Source: CAD feature listing. Evaluate the final solid. Frame: model axes, mm. A direction names the side the tool comes from. Round coordinates to 2 decimals unless told otherwise and drop trailing zeros. Loops run counter-clockwise (first coordinate to the right, second up) from the corner with the lowest first, then second, coordinate; pieces in that order, holes last. Notation, with made-up numbers: M -12,15 L 40,15 A23 cw 40,52 Z; hole C 13,67.5 d1. An arc over 180 degrees is marked long. Answer as a JSON object with one key per item and string values.
from build123d import *

# Parameters (mm, degrees)
ESQUISSE1_R                  = 4.1
BOSS_EXTRU_1_DEPTH           = 5
ESQUISSE2_R                  = 8.25
ENL_V_MAT_EXTRU_1_DEPTH      = 3
ESQUISSE4_W                  = 3
ESQUISSE4_H                  = 5
ENL_V_MAT_EXTRU_2_DEPTH      = 2
BOSS_EXTRU_2_DEPTH           = 5
ENL_V_MAT_EXTRU_4_DEPTH      = 5
ESQUISSE8_R                  = 2.75
ENL_V_MAT_EXTRU_5_DEPTH      = 6
ENL_V_MAT_EXTRU_5_DEPTH_BACK = 6


with BuildPart() as part:
    # Esquisse1 → Boss.-Extru.1 (new body)
    with BuildSketch(Plane.XY):
        with BuildLine():
            Line((-11, -4.795831523), (-4.5, -18.795831523))
            Line((-4.5, -18.795831523), (4.5, -18.795831523))
            Line((4.5, -18.795831523), (11, -4.795831523))
            ThreePointArc((11, -4.795831523), (0, 12), (-11, -4.795831523))
        make_face()
        Circle(ESQUISSE1_R, mode=Mode.SUBTRACT)
    extrude(amount=BOSS_EXTRU_1_DEPTH)

    # Esquisse2 → Enlèv. mat.-Extru.1 (cut)
    with BuildSketch(Plane.XY.offset(5)):
        Circle(ESQUISSE2_R)
    extrude(amount=-ENL_V_MAT_EXTRU_1_DEPTH, mode=Mode.SUBTRACT)

    # Esquisse4 → Enlèv. mat.-Extru.2 (cut)
    with BuildSketch(Plane(origin=(0, 12, 0), x_dir=(1, 0, 0), z_dir=(0, 1, 0))):
        with Locations((0, -2.5)):
            Rectangle(ESQUISSE4_W, ESQUISSE4_H)
    extrude(amount=-ENL_V_MAT_EXTRU_2_DEPTH, mode=Mode.SUBTRACT)

    # Esquisse6 → Boss.-Extru.2 (add)
    with BuildSketch(Plane.XY.offset(5)):
        Polygon((0, -18.795831523), (4.5, -18.795831523), (7.75, -11.795831523), (0, -11.795831523), align=None)
    extrude(amount=BOSS_EXTRU_2_DEPTH)

    # Esquisse7 → Enlèv. mat.-Extru.4 (cut)
    with BuildSketch(Plane.XY.offset(5)):
        Polygon((0, -18.795831523), (0, -11.795831523), (-7.75, -11.795831523), (-4.5, -18.795831523), align=None)
    extrude(amount=-ENL_V_MAT_EXTRU_4_DEPTH, mode=Mode.SUBTRACT)

    # Esquisse8 → Enlèv. mat.-Extru.5 (cut, two sides)
    with BuildSketch(Plane.XY.offset(5)) as enl_v_mat_extru_5_sk:
        with Locations((0, -13)):
            Circle(ESQUISSE8_R)
    extrude(amount=ENL_V_MAT_EXTRU_5_DEPTH, mode=Mode.SUBTRACT)
    extrude(enl_v_mat_extru_5_sk.sketch, amount=-ENL_V_MAT_EXTRU_5_DEPTH_BACK, mode=Mode.SUBTRACT)


solid = part.part
Item 1: Section D-D on x = 2. Return the cut outline in (y, z), then the cut area to 3 significant figures.
Answer sheet:
{"outline": "M -18.8,0 L -14.89,0 L -14.89,10 L -18.8,10 Z; M -11.11,0 L -3.58,0 L -3.58,2 L -8,2 L -8,5 L -11.11,5 Z; M 3.58,0 L 11.83,0 L 11.83,5 L 8,5 L 8,2 L 3.58,2 Z", "area": "91.5 mm²"}
Item 2: Contact query for flat-ended pins moving along their axis: pin 1 Ø0.9 at (x, z) = (0, 2.5) entering from +Y; pin 2 Ø0.9 at (y, z) = (-17.5, 6.5) entering from -X; pin 3 Ø5 at (x, y) = (0, -13) entering from +Z; pin 4 Ø3 at (x, z) = (-5, 2) entering from -Y. Output: stop coordinate, or through.
Answer sheet:
{"pin 1": "stops at y = 10", "pin 2": "stops at x = 0", "pin 3": "passes through", "pin 4": "stops at y = -11.8"}
Item 3: Section A-A on z = 1. Return the cut outline in (x, y).
Answer sheet:
{"outline": "M -11,-4.8 L -7.75,-11.8 L -2.47,-11.8 A2.75 cw long 0,-15.75 L 0,-18.8 L 4.5,-18.8 L 11,-4.8 A12 ccw 1.5,11.91 L 1.5,10 L -1.5,10 L -1.5,11.91 A12 ccw Z; hole C 0,0 d8.2"}
Item 4: Section C-C on z = 6.25. Return the cut outline in (x, y), then the cut area to 3 significant figures.
Answer sheet:
{"outline": "M 0,-18.8 L 4.5,-18.8 L 7.75,-11.8 L 2.47,-11.8 A2.75 cw 0,-15.75 Z", "area": "33.7 mm²"}
Item 5: Line query: probe 1 along X at (y, z) = (0, 1.5); probe 2 along Y at (x, z) = (0.5, 3.75); probe 3 along Z at (x, y) = (0, 6). Output: solid intervals per line, ascending. Write a range as from..to.
Answer sheet:
{"probe 1": "x = -12..-4.1, 4.1..12", "probe 2": "y = -18.8..-15.7, -10.3..-8.23, 8.23..10", "probe 3": "z = 0..2"}
Item 6: Section B-B on y = 0.5. Return the cut outline in (x, z).
Answer sheet:
{"outline": "M -11.99,0 L -4.07,0 L -4.07,2 L -8.23,2 L -8.23,5 L -11.99,5 Z; M 4.07,0 L 11.99,0 L 11.99,5 L 8.23,5 L 8.23,2 L 4.07,2 Z"}
Item 7: Pull-direction query (X, two-part tool) for faces 1 (the cylindrical face through (2.746, -12.847, 3.959)), 2 (the flat face through (8, 3, 5)), 3 (the flat face through (6.98, -13.45, 3.82)), 4 (the flat face through (0, -17, 5)); classes: pulls with the +X half, pulls with the -X half, needs draft (parallel to the pull), parting line crosses it, or undercut.
Answer sheet:
{"face 1": "undercut", "face 2": "needs draft", "face 3": "pulls with the +X half", "face 4": "pulls with the -X half"}
Item 8: Access query for faces 5 (the cylindrical face through (7.62, -3.16, 3.52)), 6 (the flat face through (5, -11.796, 7)), 7 (the flat face through (1.5, 11, 3)). Directions: +Z, -Z, +X, -X, +Y, -Y. A direction counts if a zero-diameter tool reaches every point of the face in a straight line with its end or side. Return the directions, or none.
Answer sheet:
{"face 5": "+Z", "face 6": "+Z, +X, -X, +Y", "face 7": "+Z, -Z, +Y"}
